The model under review builds one solid part; all positions refer to its coordinate system, in mm. Face numbers are marked on the shaded views. A direction names the side the tool comes from. Coordinates: 2 decimals unless noted, no trailing zeros. Write each loop counter-clockwise with the first axis right and the second up, starting at its lowest first coordinate (ties: lowest second). Pieces come first, ordered by that corner, then holes.
1) For line 1 (X direction, y = 1.3, z = 4); line 2 (X direction, y = 0.7, z = 3.5); line 3 (X direction, y = 1.35, z = -1.75), list the stretches that pass through material, from the lowest coordinate up.
2) Mouldability with a two-part tool opening along X and no side actions: class the marked faces 5, 6 and 7 as released by +X, released by -X, zero draft, split by the parting line, or undercut.
3) Machinability: for the marked faces 1, 2, 3 and 4, which of the approach directions +Z, -Z, +X, -X, +Y, -Y give a long, thin tool a straight path to every point of the face, cutting with its end or side? Answer none if there is none.
4) Add section B-B, the plane y = 1.65. State the section outline as (x, z) points, then the cut area to 3 significant figures.
5) For P1, Ø2, axis at x = 11.5, z = -5.5, coming from the +Y side; P2, Ø6, axis at x = 10, z = -1.5, coming from the +Y side; P3, Ø1.4, axis at x = 8.58, z = 4, coming from the +Y side, all flat-tipped, find the tip position at first contact; note any pin that passes through.
6) Add section D-D, the plane z = 0.75. State the section outline as (x, y) points.
7) Add section A-A, the plane z = -2. State the section outline as (x, y) points.
8) Add section C-C, the plane x = 10. State the section outline as (y, z) points.
from build123d import *

# Parameters (mm, degrees)
MAINBASESKETCH_W        = 15.8
MAINBASESKETCH_H        = 3.2
MAINBASEEXTRUDE_DEPTH   = 7.9
STUDSSKETCH_R           = 2.4
STUDSEXTRUDE_DEPTH      = 1.6
STUDSPATTERN_COUNT      = 2
STUDSPATTERN_PITCH      = 8
STUDSPATTERN_COUNT_DIR2 = 2
STUDSPATTERN_PITCH_DIR2 = 8
MAINBASESHELL_T         = -1.2
LCUTBLUE_DEPTH          = 19.555463972
LCUTBLUE_DEPTH_BACK     = 19.555463972
MADESLIMCUTSKETCH_W     = 7.9
MADESLIMCUTSKETCH_H     = 7.9
MADESLIMCUT_DEPTH       = 19.897228453
SLIMHOLEEXT_START       = -0.2
SLIMHOLESKETCH_R        = 1.75
SLIMHOLESKETCH_R_2      = 0.75
SLIMHOLEEXT_DEPTH       = 2
BOSS_EXTRUDE2_DEPTH     = 2.5
SKETCH80_R              = 1.653025405
BOSS_EXTRUDE3_DEPTH     = 14


with BuildPart() as part:
    # MainBaseSketch → MainBaseExtrude (new, symmetric)
    with BuildSketch(Plane.XY):
        with Locations((8.581967213, 1.6)):
            Rectangle(MAINBASESKETCH_W, MAINBASESKETCH_H)
    extrude(amount=MAINBASEEXTRUDE_DEPTH, both=True)

    # StudsSketch → StudsExtrude (add)
    with BuildSketch(Plane(origin=(0, 3.2, 0), x_dir=(1, 0, 0), z_dir=(0, 1, 0))):
        with Locations((4.581967213, 4)):
            Circle(STUDSSKETCH_R)
    studsextrude = extrude(amount=STUDSEXTRUDE_DEPTH)

    # StudsPattern: StudsExtrude 2 × 2
    with Locations(*[(j * STUDSPATTERN_PITCH_DIR2, 0, i * STUDSPATTERN_PITCH) for i in range(STUDSPATTERN_COUNT) for j in range(STUDSPATTERN_COUNT_DIR2) if (i, j) != (0, 0)]):
        add(studsextrude)

    # MainBaseShell
    mainbaseshell_openings = [part.faces().sort_by_distance(p)[0] for p in [
        (8.581967213, 0, 0),
    ]]
    offset(amount=MAINBASESHELL_T, openings=mainbaseshell_openings, kind=Kind.INTERSECTION)

    # LCUTBlueSketch → LCutBlue (cut, two sides: drawn at the far end of the back side and taken through both)
    with BuildSketch(Plane(origin=(0, 3.2, 0), x_dir=(1, 0, 0), z_dir=(0, 1, 0)).offset(-LCUTBLUE_DEPTH_BACK)):
        Polygon((8.581967213, 53.229874044), (8.581967213, 7.9), (8.581967213, 0), (16.481967213, 0), (61.811841258, 0), (125.917963912, 64.106122654), (72.688089868, 117.335996699), align=None)
    extrude(amount=LCUTBLUE_DEPTH + LCUTBLUE_DEPTH_BACK, mode=Mode.SUBTRACT)

    # MadeSlimCutSketch → MadeSlimCut (cut, through all)
    with BuildSketch(Plane.XZ):
        with Locations((4.631967213, -3.95)):
            Rectangle(MADESLIMCUTSKETCH_W, MADESLIMCUTSKETCH_H)
    extrude(amount=-MADESLIMCUT_DEPTH, mode=Mode.SUBTRACT)

    # SlimHoleSketch → SlimHoleExt (add)
    with BuildSketch(Plane.XZ.offset(-2).offset(SLIMHOLEEXT_START)):
        with Locations((8.581967213, 4)):
            Circle(SLIMHOLESKETCH_R)
        with Locations((8.581967213, 4)):
            Circle(SLIMHOLESKETCH_R_2, mode=Mode.SUBTRACT)
    extrude(amount=SLIMHOLEEXT_DEPTH)

    # Sketch78 → Boss-Extrude2 (add)
    with BuildSketch(Plane.ZY.offset(-0.681967213)):
        with BuildLine():
            Line((0, 0), (-4.9, 0))
            ThreePointArc((-4.9, 0), (-6.859591794, 3.785640646), (-2.6372583, 3.2))
            Line((-2.6372583, 3.2), (0, 3.2))
            Line((0, 3.2), (0, 0))
        make_face()
    boss_extrude2 = extrude(amount=-BOSS_EXTRUDE2_DEPTH)

    # Mirror9: Boss-Extrude2 across plane
    add(boss_extrude2.mirror(Plane.ZY.offset(-8.581967213)))

    # Sketch80 → Boss-Extrude3 (add)
    with BuildSketch(Plane.ZY.offset(-0.681967213)):
        with Locations((-4.9, 2.4)):
            Circle(SKETCH80_R)
    extrude(amount=-BOSS_EXTRUDE3_DEPTH)


solid = part.part
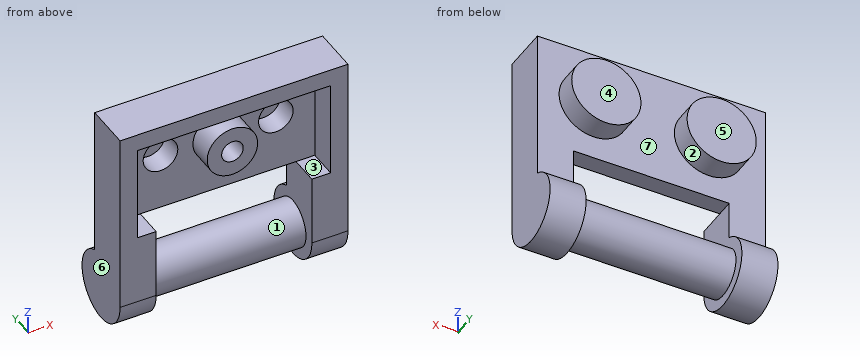
Geometry results:
1. line 1: x = 0.68 to 1.88, 6.83 to 7.83, 9.33 to 10.33, 15.28 to 16.48
1. line 2: x = 0.68 to 1.88, 6.9 to 8.02, 9.14 to 10.26, 15.28 to 16.48
1. line 3: x = 0.68 to 3.18, 13.98 to 16.48
2. face 5: zero draft
2. face 6: released by -X
2. face 7: undercut
3. face 1: none
3. face 2: +Y
3. face 3: -Y
3. face 4: +Z, -Z, +X, -X, +Y
4. outline: (0.68, -7.18) - (3.18, -7.18) - (3.18, -6.37) - (13.98, -6.37) - (13.98, -7.18) - (16.48, -7.18) - (16.48, 7.9) - (0.68, 7.9) - close; circle Ø3.5 at (8.58, 4); hole (1.88, 0) - (3.18, 0) - (3.18, -3.43) - (13.98, -3.43) - (13.98, 0) - (15.28, 0) - (15.28, 6.7) - (1.88, 6.7) - close; hole circle Ø1.5 at (8.58, 4)
4. area: 111 mm2
5. P1: stops at y = 4.05
5. P2: stops at y = 4
5. P3: stops at y = 3.2
6. outline: (0.68, 0) - (1.88, 0) - (1.88, 2) - (15.28, 2) - (15.28, 0) - (16.48, 0) - (16.48, 3.2) - (0.68, 3.2) - close
7. outline: (0.68, 0) - (3.18, 0) - (3.18, 3.2) - (0.68, 3.2) - close; (13.98, 0) - (16.48, 0) - (16.48, 3.2) - (13.98, 3.2) - close
8. outline: (0, 6.7) - (2, 6.7) - (2, 5.03) - (0.2, 5.03) - (0.2, 2.97) - (2, 2.97) - (2, 0) - (3.2, 0) - (3.2, 7.9) - (0, 7.9) - close; circle Ø3.31 at (2.4, -4.9)
